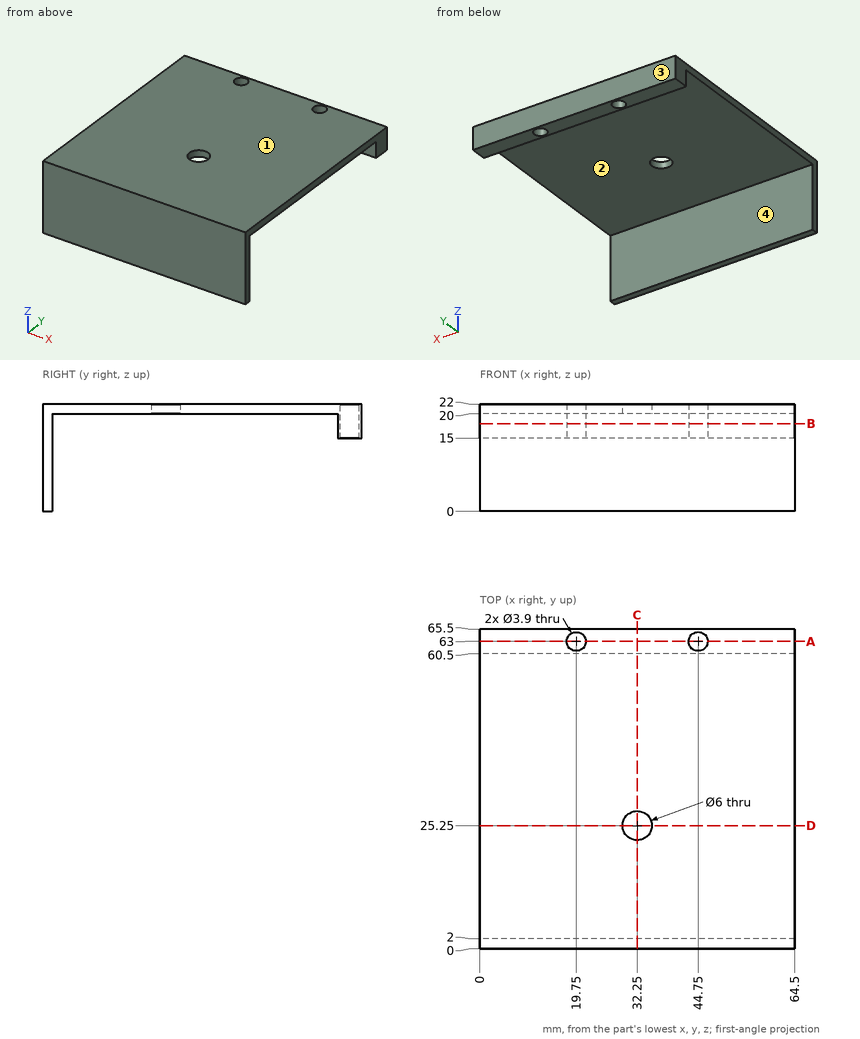
Verification items for this drawing (mm, ordinates from the low corner). Round coordinates to 2 decimals unless told otherwise and drop trailing zeros. Loops run counter-clockwise (first coordinate to the right, second up) from the corner with the lowest first, then second, coordinate; pieces in that order, holes last. Notation, with made-up numbers: (59, -18) - (86, -18) arc R15 ccw to (86, -7) - close; hole circle Ø3 at (-40, 16). An arc over 180 degrees is marked (long way). Write item = value, one per line.
Q1. Depth check by flat-ended pin: pin 1 (4.5 mm diameter, centred on x = 19.75, y = 63, fed in from +Z); pin 2 (9.5 mm diameter, centred on x = 32.25, y = 25.25, fed in from -Z); pin 3 (12 mm diameter, centred on x = 37.5, z = 5, fed in from +Y); pin 4 (2.5 mm diameter, centred on x = 20.5, y = 63.5, fed in from -Z). Enter the tip coordinate at first touch or a pass-through.
Here are the results:
pin_1 = 22
pin_2 = 20
pin_3 = 2
pin_4 = 15
Q2. Mould release check, pull along Y, two halves, no side actions. Record for the marked faces 1, 2, 3 and 4: +Y half, -Y half, draft (parallel to the pull), parting line (faces both ways), or undercut.
Here are the results:
face_1 = draft
face_2 = undercut
face_3 = +Y half
face_4 = undercut
Q3. Sectioned sample at D-D on y = 25.25. Record the boundary of the cut face in (x, z).
Here are the results:
outline = (0, 20) - (29.25, 20) - (29.25, 22) - (0, 22) - close; (35.25, 20) - (64.5, 20) - (64.5, 22) - (35.25, 22) - close
Q4. Sectioned sample at B-B on z = 18. Record the boundary of the cut face in (x, y).
Here are the results:
outline = (0, 0) - (64.5, 0) - (64.5, 2) - (0, 2) - close; (0, 60.5) - (64.5, 60.5) - (64.5, 65.5) - (0, 65.5) - close; hole circle Ø3.9 at (19.75, 63); hole circle Ø3.9 at (44.75, 63)
Q5. Material ranges on L1, parallel to X at y = 63, z = 16.5; L2, parallel to Y at x = 32.25, z = 20.8; L3, parallel to Y at x = 3.5, z = 16.25, recorded low to high.
Here are the results:
L1 = 0 to 17.8, 21.7 to 42.8, 46.7 to 64.5
L2 = 0 to 22.25, 28.25 to 65.5
L3 = 0 to 2, 60.5 to 65.5
Q6. Sectioned sample at C-C on x = 32.25. Record the boundary of the cut face in (y, z), plus the area to 3 significant figures.
Here are the results:
outline = (0, 0) - (2, 0) - (2, 20) - (22.25, 20) - (22.25, 22) - (0, 22) - close; (28.25, 20) - (60.5, 20) - (60.5, 15) - (65.5, 15) - (65.5, 22) - (28.25, 22) - close
area = 184 mm^2
Q7. Sectioned sample at A-A on y = 63. Record the boundary of the cut face in (x, z), plus the area to 3 significant figures.
Here are the results:
outline = (0, 15) - (17.8, 15) - (17.8, 22) - (0, 22) - close; (21.7, 15) - (42.8, 15) - (42.8, 22) - (21.7, 22) - close; (46.7, 15) - (64.5, 15) - (64.5, 22) - (46.7, 22) - close
area = 397 mm^2
